Build history of the part. All positions in model axes, mm. A direction names the side the tool comes from. Coordinates: 2 decimals unless noted, no trailing zeros. Loops run counter-clockwise (first coordinate to the right, second up) from the corner with the lowest first, then second, coordinate; pieces in that order, holes last. Notation, with made-up numbers: (86, 83.25) - (142, 83.25) arc R30 cw to (142, 116.25) - close; hole circle Ø2 at (80, 23). An arc over 180 degrees is marked (long way). One line per item, written item: value.
Autodesk Fusion 360 part; units mm, degrees
sketch "Sketch1" plane through (0, 0, 0) normal (0, 1, 0) x (1, 0, 0)
  circle A0 centre (10, -10) radius 2.25
  line L0 (-3, 3) -> (22, 3)
  line L1 (-3, 3) -> (-3, -22)
  line L2 (0, 0) -> (22, 0)
  line L3 (22, 0) -> (22, -22)
  line L4 (22, -22) -> (0, -22)
  line L5 (0, -22) -> (0, 0)
  line L6 (22, 3) -> (22, 0)
  line L7 (-3, -22) -> (0, -22)
  dimension "d1" = 4.5
  dimension "d2" = 10
  dimension "d3" = 10
  dimension "d4" = 3
  dimension "d5" = 3
  dimension "d6" = 22
  dimension "d7" = 22
  dimension "d8" = 25
  dimension "d9" = 25
extrude "Extrude1" add sketch "Sketch1" along normal blind 6 contours L0 L1 L2 L5 L6 L7
extrude "Extrude2" add sketch "Sketch1" against normal blind 3.2
chamfer "Chamfer1" distance 1.6 angle 45 1 edges at (-3, 1.4, -3)
fillet "Fillet1" radius 12 1 edges at (22, -1.6, 22)
sketch "Sketch2" plane through (0, -3.2, 0) normal (0, -1, 0) x (1, 0, 0)
  circle A0 centre (10, 10) radius 2.25
  arc A1 (22, 10) -> (10, 22) centre (10, 10) ccw
  line L0 (10, 22) -> (-3, 22)
  line L1 (-3, 22) -> (-3, -1.4)
  line L2 (-3, -1.4) -> (-1.4, -3)
  line L3 (-1.4, -3) -> (22, -3)
  line L4 (22, -3) -> (22, 10)
  circle A2 centre (10, 10) radius 2.25
  line L5 (10, 5.9585) -> (13.5, 7.9793)
  line L6 (13.5, 7.9793) -> (13.5, 12.0207)
  line L7 (13.5, 12.0207) -> (10, 14.0415)
  line L8 (10, 14.0415) -> (6.5, 12.0207)
  line L9 (6.5, 12.0207) -> (6.5, 7.9793)
  line L10 (6.5, 7.9793) -> (10, 5.9585)
  point P0 (10, 10)
  dimension "d17" = 3.5
extrude "Extrude3" add sketch "Sketch2" along normal blind 3.4 contours A1 L0 L1 L2 L3 L4
sketch "Sketch3" plane through (0, -3.2, 0) normal (0, -1, 0) x (1, 0, 0)
  line L0 (10, 5.9585) -> (13.5, 7.9793)
  line L1 (13.5, 7.9793) -> (13.5, 12.0207)
  line L2 (13.5, 12.0207) -> (10, 14.0415)
  line L3 (10, 14.0415) -> (6.5, 12.0207)
  line L4 (6.5, 12.0207) -> (6.5, 7.9793)
  line L5 (6.5, 7.9793) -> (10, 5.9585)
  circle A0 centre (10, 10) radius 2.25
  line L6 (9.6029, 6.1878) -> (6.5, 11.5622)
  line L7 (13.5, 8.4378) -> (10.3971, 13.8122)
  line L8 (13.1029, 7.75) -> (6.8971, 7.75)
  line L9 (13.1029, 12.25) -> (6.8971, 12.25)
  circle A1 centre (10, 10) radius 2.25
extrude "Extrude4" cut sketch "Sketch3" against normal blind 0.4 contours L0 L1 A0 L7 L8 A1 | A0 L6 L8 A1 | L3 L4 A0 L6 L9 A1 | A0 L7 L9 A1
extrude "Extrude5" cut sketch "Sketch3" against normal blind 0.2 contours L0 L5 L6 L8 | L2 L3 L7 L9
chamfer "Chamfer2" distance 0.4 angle 45 1 faces at (0.1667, -6.6, 10.8736)
equation "d17 = ( 7 / 2 ) * 1 mm"
Item 1: Cut at A-A, the plane y = -4.75. Write the cut outline in (x, z).
Check result:
outline: (-3, -1.4) - (-1.4, -3) - (22, -3) - (22, 10) arc R12 ccw to (10, 22) - (-3, 22) - close; hole (6.5, 7.98) - (10, 5.96) - (13.5, 7.98) - (13.5, 12.02) - (10, 14.04) - (6.5, 12.02) - close
Item 2: Drop flat-ended pins along their axis: P1, Ø1.5, axis at y = -3, z = 18, coming from the +X side; P2, Ø6.5, axis at x = 13.5, z = 9, coming from the +Y side; P3, Ø0.9, axis at x = 12, z = 7, coming from the -Y side; P4, Ø2.5, axis at x = 12, z = 10.5, coming from the -Y side. Give the stop position or say it passes through.
Check result:
P1: stops at x = 19.56
P2: stops at y = 0
P3: stops at y = -6.6
P4: stops at y = -3.2
Item 3: Tool access for faces 1 (the face through (8.8, -2.8, 7.9)), 2 (the face through (22, -1, 2)): list every direction of +Z, -Z, +X, -X, +Y, -Y with a clear straight run to the whole face (end or side of a thin tool).
Check result:
face 1: -Y
face 2: +Z, -Z, +X, +Y, -Y
Item 4: Pull direction Z, two halves, no side cores. Call faces 3 (the face through (6.5, -4, 10)), 4 (the face through (7, -6.6, 7)), 5 (the face through (10, 0, -3)), 6 (the face through (10, -3, 7)): released by +Z, released by -Z, zero draft, split by the parting line, or undercut.
Check result:
face 3: undercut
face 4: zero draft
face 5: released by -Z
face 6: undercut
Item 5: Cut at B-B, the plane x = 0.5. Write the cut outline in (y, z), then the cut area to 3 significant figures.
Check result:
outline: (-6.6, -2.6) - (-6.2, -3) - (6, -3) - (6, 0) - (0, 0) - (0, 22) - (-6.2, 22) - (-6.6, 21.6) - close
area: 183 mm^2
Item 6: Probe probe 1 along X at (y, z) = (-1.65, 10); probe 2 along Y at (x, z) = (13, 14.5). List the from-to ranges inside material, lowest first. Write a range as from..to.
Check result:
probe 1: x = -3..7.75, 12.25..22
probe 2: y = -6.6..0
